from build123d import *

# Parameters (mm, degrees)
PAD_DEPTH    = 3
POCKET_DEPTH = 3.001


with BuildPart() as part:
    # Sketch → Pad (new body)
    with BuildSketch(Plane.XY):
        with BuildLine():
            Line((0, 11.045), (10, 11.045))
            ThreePointArc((15, 6.045), (13.535534, 9.580534), (10, 11.045))
            Line((15, 6.045), (15, -6.045))
            ThreePointArc((10, -11.045), (13.535534, -9.580534), (15, -6.045))
            Line((10, -11.045), (0, -11.045))
            Line((0, -11.045), (0, 11.045))
        make_face()
    extrude(amount=PAD_DEPTH)

    # Sketch001 → Pocket (cut, through all)
    with BuildSketch(Plane.XY):
        with BuildLine():
            Line((1.860247, 8.045), (8.695431, 8.045))
            ThreePointArc((13.695431, 3.045), (12.230965, 6.580534), (8.695431, 8.045))
            Line((13.695431, 3.045), (13.695431, -4.201112))
            ThreePointArc((8.695431, -9.201112), (12.230965, -7.736646), (13.695431, -4.201112))
            Line((8.695431, -9.201112), (1.860247, -9.201112))
            Line((1.860247, -9.201112), (1.860247, 8.045))
        make_face()
    extrude(amount=POCKET_DEPTH, mode=Mode.SUBTRACT)


solid = part.part
Part model, mm, in its own coordinate system. A direction names the side the tool comes from. Coordinates: 2 decimals unless noted, no trailing zeros. Order: outer loops, then holes, each group sorted by start corner. A loop starts at its lowest first (then second) coordinate and runs counter-clockwise, first axis right, second up.
(1) Pin check, flat tip, straight feed: pin 1 Ø0.9 at (y, z) = (-2, 2) entering from -X. Stop position of the tip, or through.
Check sheet entries:
pin 1: stops at x = 0
(2) Slice it at B-B, the plane x = 5.25. Write the cut outline in (y, z) (3 decimals), and give its area (3 significant figures).
Check sheet entries:
outline: (-11.045, 0) - (-9.201, 0) - (-9.201, 3) - (-11.045, 3) - close; (8.045, 0) - (11.045, 0) - (11.045, 3) - (8.045, 3) - close
area: 14.5 mm2
(3) Tool access for faces 4 (the face through (5, -9.201, 1)), 5 (the face through (5, -11.045, 1)): list every direction of +Z, -Z, +X, -X, +Y, -Y with a clear straight run to the whole face (end or side of a thin tool).
Check sheet entries:
face 4: +Z, -Z
face 5: +Z, -Z, +X, -X, -Y
(4) Pull direction X, two halves, no side cores. Call faces 1 (the face through (13.695, -1, 1)), 2 (the face through (0, 0, 1)), 3 (the face through (1, 0, 3)): pulls with the +X half, pulls with the -X half, needs draft (parallel to the pull), parting line crosses it, or undercut.
Check sheet entries:
face 1: undercut
face 2: pulls with the -X half
face 3: needs draft
(5) Probe L1, parallel to X at y = -0.75, z = 2.1; L2, parallel to Y at x = 3.5, z = 1.45 (3 decimals); L3, parallel to X at y = 6.25, z = 1.9. List the from-to ranges inside material, lowest first.
Check sheet entries:
L1: x = 0 to 1.86, 13.7 to 15
L2: y = -11.045 to -9.201, 8.045 to 11.045
L3: x = 0 to 1.86, 12.53 to 15
(6) Slice it at A-A, the plane y = 2.5. Write the cut outline in (x, z).
Check sheet entries:
outline: (0, 0) - (1.86, 0) - (1.86, 3) - (0, 3) - close; (13.7, 0) - (15, 0) - (15, 3) - (13.7, 3) - close
(7) Slice it at C-C, the plane z = 2.35. Write the cut outline in (x, y) (3 decimals), and give its area (3 significant figures).
Check sheet entries:
outline: (0, -11.045) - (10, -11.045) arc R5 ccw to (15, -6.045) - (15, 6.045) arc R5 ccw to (10, 11.045) - (0, 11.045) - close; hole (1.86, -9.201) - (8.695, -9.201) arc R5 ccw to (13.695, -4.201) - (13.695, 3.045) arc R5 ccw to (8.695, 8.045) - (1.86, 8.045) - close
area: 127 mm2
